from build123d import *

# Parameters (mm, degrees)
F1_DEPTH = 38.1
F0_W     = 18.215902
F0_H     = 19.05
F2_DEPTH = 15.875
F4_R     = 12.7


with BuildPart() as f1:
    # F0 (on Front) → F1 (new body, symmetric)
    with BuildSketch(Plane.XZ):
        Polygon((-41.398831, -9.801595), (41.398831, -9.801595), (41.398831, 9.801595), (22.34883, 9.801595), (-41.398831, 9.801595), align=None)
    extrude(amount=F1_DEPTH, both=True)

    # F0 (on Front) → F2 (join, symmetric)
    with BuildSketch(Plane.XZ):
        with BuildLine():
            Line((22.34883, 9.801595), (41.398831, 9.801595))
            Line((41.398831, 9.801595), (41.398831, 38.174614))
            ThreePointArc((41.398831, 38.174614), (43.258703, 42.664742), (47.74883, 44.524614))
            Line((47.74883, 44.524614), (69.194875, 44.524614))
            Line((69.194875, 44.524614), (69.194875, 63.574614))
            Line((69.194875, 63.574614), (47.74883, 63.574614))
            ThreePointArc((47.74883, 63.574614), (29.788318, 56.135127), (22.34883, 38.174614))
            Line((22.34883, 38.174614), (22.34883, 9.801595))
        make_face()
        with Locations((78.302826, 54.049614)):
            Rectangle(F0_W, F0_H)
    extrude(amount=F2_DEPTH, both=True)

    # F0 (on Front) → F3 (revolve)
    with BuildSketch(Plane.XZ):
        Polygon((87.410777, 44.524614), (69.194875, 44.524614), (69.194875, 36.908722), (94.594875, 36.908722), (94.594875, 69.924614), (69.194875, 69.924614), (69.194875, 63.574614), (87.410777, 63.574614), align=None)
    revolve(axis=Axis((69.194875, 0, 53.416668), (0, 0, 1)))

    # F4
    f4_edges = [f1.edges().sort_by_distance(p)[0] for p in [
        (-41.398831, -38.1, 0),
        (41.398831, -38.1, 0),
        (-41.398831, 38.1, 0),
        (41.398831, 38.1, 0),
    ]]
    fillet(f4_edges, radius=F4_R)


solid = f1.part
Read the model definition and answer for the solid it produces. Units are mm, in the model's axes. A direction names the side the tool comes from. Give positions to 0.01 mm unless a question says otherwise; leave off trailing zeros. Loops run counter-clockwise (first coordinate to the right, second up) from the corner with the lowest first, then second, coordinate; pieces in that order, holes last. Notation, with made-up numbers: (39, -1) -> (70, -1) arc R24 ccw to (70, 10) -> close; hole circle Ø2 at (68, -11.5). An arc over 180 degrees is marked (long way). Use a Markdown table: item, result.
Q1. Section B-B, the plane x = 36.5 is taken. Determine the outline of the cut face in (y, z) (3 decimals).
Solved:
| item | result |
|---|---|
| outline | (-35.422, -9.802) -> (35.422, -9.802) -> (35.422, 9.802) -> (15.875, 9.802) -> (15.875, 60.948) -> (-15.875, 60.948) -> (-15.875, 9.802) -> (-35.422, 9.802) -> close |
Q2. Section C-C, the plane z = 40.5 is taken. Determine the outline of the cut face in (x, y) (1 decimal).
Solved:
| item | result |
|---|---|
| outline | (22.5, -15.9) -> (41.8, -15.9) -> (41.8, 15.9) -> (22.5, 15.9) -> close; circle Ø50.8 at (69.2, 0) |
Q3. Find the intervals of material crossed by line 1 along Z through (x, y) = (82, 10); line 2 along Z through (x, y) = (24, 26); line 3 along Y through (x, z) = (23.5, 42) (3 decimals), in increasing order.
Solved:
| item | result |
|---|---|
| line 1 | z = 36.91 to 69.92 |
| line 2 | z = -9.8 to 9.8 |
| line 3 | y = -15.875 to 15.875 |
Q4. Section A-A, the plane y = -22 is taken. Determine the outline of the cut face in (x, z).
Solved:
| item | result |
|---|---|
| outline | (-41.4, -9.8) -> (41.4, -9.8) -> (41.4, 9.8) -> (-41.4, 9.8) -> close; (56.5, 36.91) -> (81.89, 36.91) -> (81.89, 69.92) -> (56.5, 69.92) -> close |
Q5. Each of these flat-tipped pins is pushed along its axis until it touches: pin 1 (8 mm diameter, centred on y = 15.5, z = 50, fed in from +X); pin 2 (3 mm diameter, centred on x = 71, z = 35.5, fed in from +Y); pin 3 (5.5 mm diameter, centred on x = 73, z = 57, fed in from -Y). Where does it stop, or does it pass through?
Solved:
| item | result |
|---|---|
| pin 1 | stops at x = 91.84 |
| pin 2 | stops at y = 25.37 |
| pin 3 | stops at y = -25.38 |
Q6. Determine the mould class of faces 1 (the face through (69, -15.875, 54)), 2 (the face through (1, -1, 9.802)), 3 (the face through (37.78, 34.28, 0.14)) for opening direction Y: pulls with the +Y half, pulls with the -Y half, needs draft (parallel to the pull), parting line crosses it, or undercut.
Solved:
| item | result |
|---|---|
| face 1 | undercut |
| face 2 | needs draft |
| face 3 | pulls with the +Y half |
Q7. A tool of negligible diameter and unlimited length cuts with its end or side. For faces 4 (the face through (33, -15.875, 37)), 5 (the face through (33, 15.875, 37)), 6 (the face through (70, 0, 36.909)), 7 (the face through (69.064, -18.215, 53.916)), from which of +Z, -Z, +X, -X, +Y, -Y can it reach the whole face along a straight path? Write none if from no direction.
Solved:
| item | result |
|---|---|
| face 4 | +Z, -X, -Y |
| face 5 | +Z, -X, +Y |
| face 6 | -Z, +X, +Y, -Y |
| face 7 | none |
Q8. Section D-D, the plane z = 48.5 is taken. Determine the outline of the cut face in (x, y) (3 decimals), then the cut area to 3 significant figures.
Solved:
| item | result |
|---|---|
| outline | (24.542, -15.875) -> (49.367, -15.875) arc R25.4 ccw (long way) to (49.367, 15.875) -> (24.542, 15.875) -> close; hole (60.262, -15.875) arc R18.216 ccw to (78.128, -15.875) -> close; hole (60.262, 15.875) -> (78.128, 15.875) arc R18.216 ccw to start |
| area | 2,640 mm^2 |
